Check sheet for the modelled part. Datum: model origin and axes. Units: mm. Face numbers are marked on the shaded views. A direction names the side the tool comes from. Coordinates: 2 decimals unless noted, no trailing zeros. Loops run counter-clockwise (first coordinate to the right, second up) from the corner with the lowest first, then second, coordinate; pieces in that order, holes last. Notation, with made-up numbers: M 63.25,15 L 73.25,15 A8 ccw 73.25,28 Z; hole C 3,19 d8. An arc over 180 degrees is marked long. Use CSV: the item, a comma, the result in double quotes. Start each with the question number.
(1) Section check B-B on y = -3. Record the cut outline in (x, z).
(2) Section check C-C on z = 1.5. Record the cut outline in (x, y).
(3) Section check A-A on x = -17.5. Record the cut outline in (y, z).
(4) Scan lines: line 1 (Z direction, x = 12, y = -16.5); line 2 (Z direction, x = -21, y = -24.5); line 3 (Z direction, x = -17, y = -24). Record each from-to range of solid material in increasing order.
(5) Set-up check for the marked faces 5, 6 and 7: record each of +Z, -Z, +X, -X, +Y, -Y from which the full face is reachable in a straight line by a thin tool's end or side.
(6) Go/stop test with flat-tipped pins: pin 1 Ø7.5 at (x, y) = (22.5, -13.5) entering from -Z; pin 2 Ø5 at (y, z) = (-4.5, 1) entering from +X; pin 3 Ø1 at (x, y) = (-25, -13) entering from +Z. Record where each tip stops, or that it passes through.
(7) Draft check along Z on the marked faces 1, 2, 3 and 4. Enter one of: pulls with the +Z half, pulls with the -Z half, needs draft (parallel to the pull), parting line crosses it, or undercut.
(8) Section check D-D on y = -18.75. Record the cut outline in (x, z), and give its area (3 significant figures).
from build123d import *

# Parameters (mm, degrees)
F1_DEPTH = 25.4
F2_R     = 5.08


with BuildPart() as f1:
    # F0 (on Front) → F1 (new body)
    with BuildSketch(Plane.XZ):
        with BuildLine():
            Line((-28.316792, 2.771431), (0, 31.449713))
            Line((0, 31.449713), (-3.456192, 34.862339))
            Line((-3.456192, 34.862339), (-31.034873, 6.93159))
            ThreePointArc((-31.034873, 6.93159), (-33.276866, -7.65281), (-20.122997, -14.339142))
            Line((-20.122997, -14.339142), (52.416187, -14.339142))
            Line((52.416187, -14.339142), (52.416187, -10.242244))
            Line((52.416187, -10.242244), (-20.122997, -10.242244))
            ThreePointArc((-20.122997, -10.242244), (-29.380141, -6.984451), (-28.316792, 2.771431))
        make_face()
    extrude(amount=F1_DEPTH)

    # F2
    f2_edges = [f1.edges().sort_by_distance(p)[0] for p in [
        (-1.728096, -25.4, 33.156026),
        (-1.728096, 0, 33.156026),
        (52.416187, -25.4, -12.290693),
        (52.416187, 0, -12.290693),
    ]]
    fillet(f2_edges, radius=F2_R)


solid = f1.part
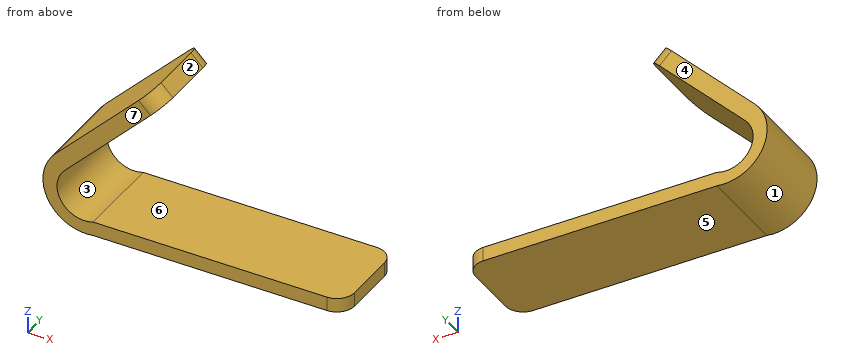
Outcome:
1,outline,"M -31.03,6.93 A12.58 ccw -20.12,-14.34 L 51.97,-14.34 L 51.97,-10.24 L -20.12,-10.24 A7.9 cw -28.32,2.77 L -0.31,31.13 L -3.77,34.55 Z"
2,outline,"M -34.19,-25.4 L -29.34,-25.4 L -29.34,0 L -34.19,0 Z"
3,outline,"M -25.4,-14.34 L 0,-14.34 L 0,-10.24 L -25.4,-10.24 Z; M -25.4,13.73 L 0,13.73 L 0,20.64 L -25.4,20.64 Z"
4,line 1,"z = -14.34 to -10.24"
4,line 2,"z = -14.45 to -10.49, 10.18 to 17.09"
4,line 3,"z = -14.34 to -10.24, 14.23 to 21.15"
5,face 5,"-Z, +X, +Y, -Y"
5,face 6,"+X, +Y, -Y"
5,face 7,"+Z, -Z, +X, -X, -Y"
6,pin 1,"stops at z = -14.34"
6,pin 2,"stops at x = -27.6"
6,pin 3,"stops at z = 13.55"
7,face 1,"parting line crosses it"
7,face 2,"pulls with the +Z half"
7,face 3,"undercut"
7,face 4,"needs draft"
8,outline,"M -31.03,6.93 A12.58 ccw -20.12,-14.34 L 52.42,-14.34 L 52.42,-10.24 L -20.12,-10.24 A7.9 cw -28.32,2.77 L 0,31.45 L -3.46,34.86 Z"
8,area,"595 mm²"
